Part model, mm, in its own coordinate system. Face numbers are marked on the shaded views. A direction names the side the tool comes from. Give positions to 0.01 mm unless a question says otherwise; leave off trailing zeros. Write each loop counter-clockwise with the first axis right and the second up, starting at its lowest first coordinate (ties: lowest second). Pieces come first, ordered by that corner, then holes. Notation, with made-up numbers: M 42,31 L 89,31 A20 cw 89,48 Z; hole C 10.25,38 d2. An arc over 180 degrees is marked long. Use CSV: the item, a comma, the result in double quotes. Start each with the question number.
Item 1: Cut at B-B (x = 33.5). List the corners of the cut face in (y, z).
Item 2: Cut at A-A (y = 0). List the corners of the cut face in (x, z) (3 decimals), then the cut area to 3 significant figures.
Item 3: Cut at C-C (y = 9.75). List the corners of the cut face in (x, z) (3 decimals).
Item 4: Which spindle directions (+Z, -Z, +X, -X, +Y, -Y) get a long thin tool onto all of the face, cutting with end or side? Do the marked faces 1 and 2. Say none if no direction does.
Item 5: Pin check, flat tips, straight feed: pin 1 (2.5 mm diameter, centred on y = -3.5, z = -2.5, fed in from -X) (3 decimals); pin 2 (3 mm diameter, centred on x = 32, y = -1, fed in from +Z); pin 3 (1.5 mm diameter, centred on x = 4, y = 2.5, fed in from -Z); pin 4 (2 mm diameter, centred on y = -7.5, z = -8, fed in from -X). Stop position of each tip, or through.
Item 6: Drill centre lines: line 1 (Z direction, x = -11.5, y = -5.75) (3 decimals); line 2 (Z direction, x = 4, y = -1.5); line 3 (Y direction, x = -18, z = -9). Where is each one in solid material? Low to high. Write a range as [from, to].
Item 7: Cut at D-D (z = -13.25). List the corners of the cut face in (x, y) (3 decimals).
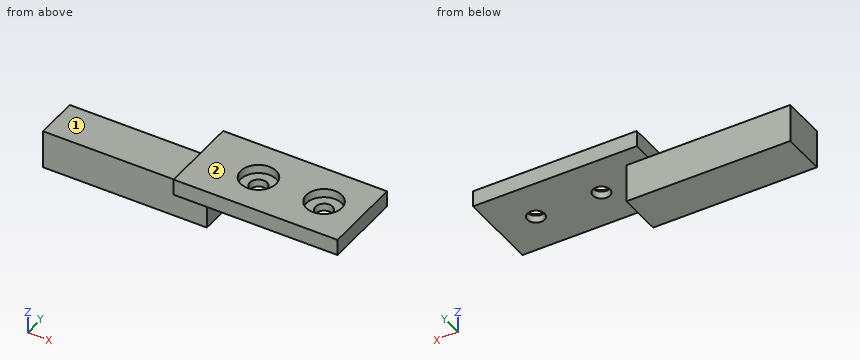
from build123d import *

# Parameters (mm, degrees)
F0_R     = 5.15874
F0_R_2   = 2.4892
F0_W     = 6.35
F0_H     = 5.3975
F0_H_2   = 12.7
F1_DEPTH = 4.699
F0_W_2   = 41.275
F2_DEPTH = 15.875
F3_DEPTH = 2.54
F4_DEPTH = 4.699


with BuildPart() as f1:
    # F0 (on Top) → F1 (new body)
    with BuildSketch(Plane.XY):
        Polygon((44.45, 11.7475), (3.175, 11.7475), (3.175, 6.35), (3.175, -6.35), (3.175, -11.7475), (44.45, -11.7475), align=None)
        with Locations((14.2875, 0)):
            Circle(F0_R, mode=Mode.SUBTRACT)
        with Locations((33.3375, 0)):
            Circle(F0_R, mode=Mode.SUBTRACT)
        with Locations((14.2875, 0)):
            Circle(F0_R)
        with Locations((14.2875, 0)):
            Circle(F0_R_2, mode=Mode.SUBTRACT)
        with Locations((33.3375, 0)):
            Circle(F0_R)
        with Locations((33.3375, 0)):
            Circle(F0_R_2, mode=Mode.SUBTRACT)
        with Locations((0, 9.04875)):
            Rectangle(F0_W, F0_H)
        Rectangle(F0_W, F0_H_2)
        with Locations((0, -9.04875)):
            Rectangle(F0_W, F0_H)
    extrude(amount=-F1_DEPTH)

    # F0 (on Top) → F2 (join)
    with BuildSketch(Plane.XY):
        with Locations((-23.8125, 0)):
            Rectangle(F0_W_2, F0_H_2)
        Rectangle(F0_W, F0_H_2)
    extrude(amount=-F2_DEPTH)

    # F0 (on Top) → F3 (cut)
    with BuildSketch(Plane.XY):
        with Locations((14.2875, 0)):
            Circle(F0_R)
        with Locations((14.2875, 0)):
            Circle(F0_R_2, mode=Mode.SUBTRACT)
        with Locations((33.3375, 0)):
            Circle(F0_R)
        with Locations((33.3375, 0)):
            Circle(F0_R_2, mode=Mode.SUBTRACT)
    extrude(amount=-F3_DEPTH, mode=Mode.SUBTRACT)

    # F0 (on Top) → F4 (cut)
    with BuildSketch(Plane.XY):
        with Locations((-23.8125, 0)):
            Rectangle(F0_W_2, F0_H_2)
    extrude(amount=-F4_DEPTH, mode=Mode.SUBTRACT)


solid = f1.part
Worked answers:
1,outline,"M -11.75,-4.7 L -2.48,-4.7 L -2.48,-2.54 L -5.16,-2.54 L -5.16,0 L -11.75,0 Z; M 2.48,-4.7 L 11.75,-4.7 L 11.75,0 L 5.16,0 L 5.16,-2.54 L 2.48,-2.54 Z"
2,outline,"M -44.45,-15.875 L 3.175,-15.875 L 3.175,-4.699 L 11.798,-4.699 L 11.798,-2.54 L 9.129,-2.54 L 9.129,0 L -3.175,0 L -3.175,-4.699 L -44.45,-4.699 Z; M 16.777,-4.699 L 30.848,-4.699 L 30.848,-2.54 L 28.179,-2.54 L 28.179,0 L 19.446,0 L 19.446,-2.54 L 16.777,-2.54 Z; M 35.827,-4.699 L 44.45,-4.699 L 44.45,0 L 38.496,0 L 38.496,-2.54 L 35.827,-2.54 Z"
2,area,"682 mm^2"
3,outline,"M -3.175,-4.699 L 44.45,-4.699 L 44.45,0 L -3.175,0 Z"
4,face 1,"+Z, -X, +Y, -Y"
4,face 2,"+Z, +X, -X, +Y, -Y"
5,pin 1,"stops at x = -3.175"
5,pin 2,"stops at z = -2.54"
5,pin 3,"stops at z = -4.7"
5,pin 4,"passes through"
6,line 1,"z = [-15.875, -4.699]"
6,line 2,"z = [-4.7, 0]"
6,line 3,"y = [-6.35, 6.35]"
7,outline,"M -44.45,-6.35 L 3.175,-6.35 L 3.175,6.35 L -44.45,6.35 Z"
